For this review, take the finished solid that the model builds, in its own axes (mm). A direction names the side the tool comes from. Coordinates: 2 decimals unless noted, no trailing zeros. Write each loop counter-clockwise with the first axis right and the second up, starting at its lowest first coordinate (ties: lowest second). Pieces come first, ordered by that corner, then holes. Notation, with made-up numbers: (30, 75.5) -> (71, 75.5) arc R27 cw to (71, 107.5) -> close; hole circle Ø10 at (41, 80.25). An arc over 180 degrees is marked (long way). One line per item, written item: value. Start each with the question number.
1) Mouldability with a two-part tool opening along Z and no side actions: class faces 1 (the cylindrical face through (10.81, 23.73, 34.34)), 2 (the flat face through (25, 0, 24)), 3 (the cylindrical face through (1.517, 20.706, 34.467)) as released by +Z, released by -Z, zero draft, split by the parting line, or undercut.
2) Machinability: for faces 4 (the flat face through (-7, 42, 0)), 5 (the flat face through (10, 5, -35)), 6 (the cylindrical face through (19.735, 43.521, 6.772)), which of the approach directions +Z, -Z, +X, -X, +Y, -Y give a long, thin tool a straight path to every point of the face, cutting with its end or side? Answer none if there is none.
3) Add section C-C (y = 14.5). State the section outline as (x, z) points, and give its area (3 significant figures).
4) For probe 1 along X at (y, z) = (42.85, 7); probe 2 along Y at (x, z) = (-35.5, -12); probe 3 along X at (y, z) = (43.5, 7), list the stretches that pass through material, from the lowest coordinate up. Write a range as from..to.
5) For pin 1 Ø3 at (x, z) = (6, 36.5) entering from -Y; pin 2 Ø6 at (x, z) = (-35, 26.5) entering from +Y; pin 3 Ø5 at (y, z) = (25, -22) entering from -X; pin 4 Ø8 at (x, y) = (32.5, 30) entering from -Z, all flat-tipped, find the tip position at first contact; note any pin that passes through.
from build123d import *

# Parameters (mm, degrees)
SKETCH1_R           = 47.5
BOSS_EXTRUDE1_DEPTH = 5
SKETCH2_R           = 36
BOSS_EXTRUDE2_DEPTH = 40
SKETCH3_R           = 34.5
CUT_EXTRUDE1_DEPTH  = 42
SKETCH4_R           = 5
CUT_EXTRUDE2_DEPTH  = 5
FILLET1_R           = 5
SKETCH5_R           = 1.75
CUT_EXTRUDE3_DEPTH  = 5
FILLET2_R           = 2


with BuildPart() as part:
    # Sketch1 → Boss-Extrude1 (new body)
    with BuildSketch(Plane(origin=(0, 0, 0), x_dir=(1, 0, 0), z_dir=(0, 1, 0))):
        with Locations(Location((0, 0, 0), (0, 0, 270))):
            Circle(SKETCH1_R)
    extrude(amount=BOSS_EXTRUDE1_DEPTH)

    # Sketch2 → Boss-Extrude2 (add)
    with BuildSketch(Plane(origin=(0, 5, 0), x_dir=(1, 0, 0), z_dir=(0, 1, 0))):
        with Locations(Location((0, 0, 0), (0, 0, 270))):
            Circle(SKETCH2_R)
    extrude(amount=BOSS_EXTRUDE2_DEPTH)

    # Sketch3 → Cut-Extrude1 (cut)
    with BuildSketch(Plane.XZ):
        with Locations(Location((0, 0, 0), (0, 0, 270))):
            Circle(SKETCH3_R)
    extrude(amount=-CUT_EXTRUDE1_DEPTH, mode=Mode.SUBTRACT)

    # Sketch4 → Cut-Extrude2 (cut)
    with BuildSketch(Plane(origin=(0, 45, 0), x_dir=(1, 0, 0), z_dir=(0, 1, 0))):
        with Locations(Location((0, 0, 0), (0, 0, 270))):
            Circle(SKETCH4_R)
    extrude(amount=-CUT_EXTRUDE2_DEPTH, mode=Mode.SUBTRACT)

    # Fillet1
    fillet1_edges = [part.edges().sort_by_distance(p)[0] for p in [
        (0, 5, -47.5),
    ]]
    fillet(fillet1_edges, radius=FILLET1_R - 0.0001)  # a hair under: the kernel refuses the full size

    # Sketch5 → Cut-Extrude3 (cut)
    with BuildSketch(Plane(origin=(0, 45, 0), x_dir=(1, 0, 0), z_dir=(0, 1, 0))):
        with Locations(Location((18, -7, 0), (0, 0, 270))):
            Circle(SKETCH5_R)
        with Locations(Location((-18, -7, 0), (0, 0, 270))):
            Circle(SKETCH5_R)
    extrude(amount=-CUT_EXTRUDE3_DEPTH, mode=Mode.SUBTRACT)

    # Fillet2
    fillet2_edges = [part.edges().sort_by_distance(p)[0] for p in [
        (0, 45, -36),
    ]]
    fillet(fillet2_edges, radius=FILLET2_R)


solid = part.part
Numbers:
1. face 1: split by the parting line
1. face 2: zero draft
1. face 3: undercut
2. face 4: -Y
2. face 5: +Y
2. face 6: +Y, -Y
3. outline: circle Ø72 at (0, 0); hole circle Ø69 at (0, 0)
3. area: 332 mm²
4. probe 1: -35.31..-19.75, -16.25..16.25, 19.75..35.31
4. probe 2: 0..5
4. probe 3: -35.25..-19.75, -16.25..16.25, 19.75..35.25
5. pin 1: y = 0
5. pin 2: y = 5
5. pin 3: x = -30.26
5. pin 4: z = -21.99
